Design review of the part built by this model. Coordinates are the model's own, in mm. Face numbers are marked on the shaded views. A direction names the side the tool comes from. Give positions to 0.01 mm unless a question says otherwise; leave off trailing zeros. Order: outer loops, then holes, each group sorted by start corner. A loop starts at its lowest first (then second) coordinate and runs counter-clockwise, first axis right, second up. Notation, with made-up numbers: (82.25, 78.5) -> (100.25, 78.5) arc R3 ccw to (100.25, 82.5) -> close; hole circle Ø2 at (-35.5, 39.5). An arc over 180 degrees is marked (long way). Answer in a Markdown table with one row per item. Add a question column.
```python
from build123d import *

# Parameters (mm, degrees)
BOSS_EXTRUDE1_DEPTH = 300
SKETCH3_W           = 50
SKETCH3_H           = 250
CUT_EXTRUDE1_DEPTH  = 20


with BuildPart() as part:
    # Sketch2 → Boss-Extrude1 (new body)
    with BuildSketch(Plane(origin=(0, 0, 0), x_dir=(0, 0, -1), z_dir=(1, 0, 0))):
        with BuildLine():
            Line((-8.879310345, 278.103448276), (-8.879310345, -26.896551724))
            Line((-8.879310345, -26.896551724), (-3.879310345, -26.896551724))
            ThreePointArc((-3.879310345, -26.896551724), (26.804536977, 125.603448276), (-3.879310345, 278.103448276))
            Line((-3.879310345, 278.103448276), (-8.879310345, 278.103448276))
        make_face()
    extrude(amount=BOSS_EXTRUDE1_DEPTH)

    # Sketch3 → Cut-Extrude1 (cut)
    with BuildSketch(Plane(origin=(0, 0, -26.804536977), x_dir=(-1, 0, 0), z_dir=(0, 0, -1))):
        with Locations((-225, 153.103448276)):
            Rectangle(SKETCH3_W, SKETCH3_H)
        with Locations((-75, 153.103448276)):
            Rectangle(SKETCH3_W, SKETCH3_H)
    extrude(amount=-CUT_EXTRUDE1_DEPTH, mode=Mode.SUBTRACT)


solid = part.part
```
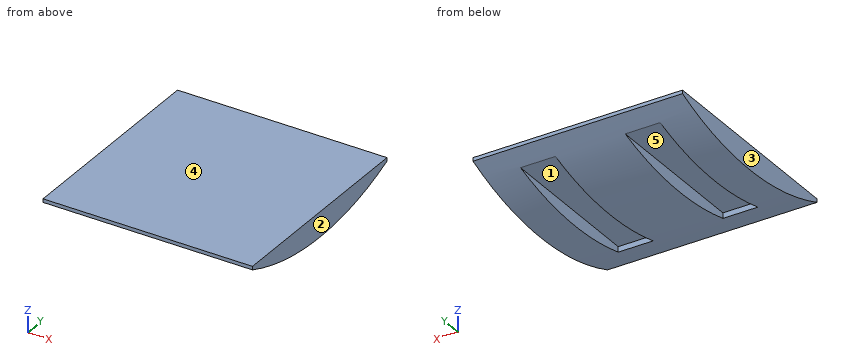
1) Machinability: for the marked faces 4 and 5, which of the approach directions +Z, -Z, +X, -X, +Y, -Y give a long, thin tool a straight path to every point of the face, cutting with its end or side? Answer none if there is none.
2) Clearance check with flat-ended pins moving along their axes: P1, Ø1.5, axis at x = 66.5, y = 171, coming from the -Z side; P2, Ø8, axis at y = 37.5, z = -2.5, coming from the -X side; P3, Ø2.5, axis at x = 73, z = -12, coming from the +Y side. State where each tip first meets the part, or that it passes through.
3) Add section D-D, the plane y = 160.5. Write out the cut boundary in (x, z), and give its area (3 significant figures).
4) Mouldability with a two-part tool opening along X and no side actions: class the marked faces 1, 2 and 3 as +X half, -X half, draft (parallel to the pull), parting line (faces both ways), or undercut.
5) Add section B-B, the plane y = 213.5. Write out the cut boundary in (x, z), and give its area (3 significant figures).
6) Add section A-A, the plane x = 236. Write out the cut boundary in (y, z), and give its area (3 significant figures).
7) Add section C-C, the plane z = -0.5. Write out the cut boundary in (x, y), and give its area (3 significant figures).
8) For L1, parallel to X at y = 130, z = -23; L2, parallel to Z at x = 212, y = 204.5; L3, parallel to Z at x = 105.5, y = 125.5, list the stretches that pass through material, from the lowest coordinate up.
Verdict:
| question | item | result |
|---|---|---|
| 1 | face 4 | +Z, +X, -X, +Y, -Y |
| 1 | face 5 | -Z, +Y |
| 2 | P1 | stops at z = -6.8 |
| 2 | P2 | stops at x = 0 |
| 2 | P3 | stops at y = 28.1 |
| 3 | outline | (0, -25.26) -> (50, -25.26) -> (50, -6.8) -> (100, -6.8) -> (100, -25.26) -> (200, -25.26) -> (200, -6.8) -> (250, -6.8) -> (250, -25.26) -> (300, -25.26) -> (300, 8.88) -> (0, 8.88) -> close |
| 3 | area | 8,400 mm2 |
| 4 | face 1 | undercut |
| 4 | face 2 | +X half |
| 4 | face 3 | -X half |
| 5 | outline | (0, -16.88) -> (50, -16.88) -> (50, -6.8) -> (100, -6.8) -> (100, -16.88) -> (200, -16.88) -> (200, -6.8) -> (250, -6.8) -> (250, -16.88) -> (300, -16.88) -> (300, 8.88) -> (0, 8.88) -> close |
| 5 | area | 6,720 mm2 |
| 6 | outline | (-26.9, 3.88) arc R394.31 ccw to (28.1, -14.56) -> (28.1, -6.8) -> (249.59, -6.8) arc R394.31 ccw to (278.1, 3.88) -> (278.1, 8.88) -> (-26.9, 8.88) -> close |
| 6 | area | 4,600 mm2 |
| 7 | outline | (0, -16) -> (300, -16) -> (300, 267.21) -> (0, 267.21) -> close |
| 7 | area | 85,000 mm2 |
| 8 | L1 | x = 0 to 50, 100 to 200, 250 to 300 |
| 8 | L2 | z = -6.8 to 8.88 |
| 8 | L3 | z = -26.8 to 8.88 |
